from build123d import *

# Parameters (mm, degrees)
SKETCH1_W           = 200
SKETCH1_H           = 5
BOSS_EXTRUDE1_DEPTH = 5
SKETCH2_W           = 4.5
SKETCH2_H           = 5
CUT_EXTRUDE1_DEPTH  = 2.475
SKETCH3_R           = 2
BOSS_EXTRUDE3_DEPTH = 4.95
SKETCH4_R           = 2
BOSS_EXTRUDE4_DEPTH = 4.95


with BuildPart() as part:
    # Sketch1 → Boss-Extrude1 (new body)
    with BuildSketch(Plane.XY):
        with Locations((100, 2.5)):
            Rectangle(SKETCH1_W, SKETCH1_H)
    extrude(amount=BOSS_EXTRUDE1_DEPTH)

    # Sketch2 → Cut-Extrude1 (cut, symmetric)
    with BuildSketch(Plane.XY.offset(2.5)):
        with Locations((2.25, 2.5)):
            Rectangle(SKETCH2_W, SKETCH2_H)
        with Locations((197.75, 2.5)):
            Rectangle(SKETCH2_W, SKETCH2_H)
    extrude(amount=CUT_EXTRUDE1_DEPTH, both=True, mode=Mode.SUBTRACT)

    # Sketch3 → Boss-Extrude3 (add)
    with BuildSketch(Plane.XY.offset(0.025)):
        with Locations(Location((2, 2.5, 0), (0, 0, 180))):
            Circle(SKETCH3_R)
    extrude(amount=BOSS_EXTRUDE3_DEPTH)

    # Sketch4 → Boss-Extrude4 (add)
    with BuildSketch(Plane.XY.offset(0.025)):
        with Locations((198, 2.5)):
            Circle(SKETCH4_R)
    extrude(amount=BOSS_EXTRUDE4_DEPTH)


solid = part.part
Geometry check sheet. Reference: the model listing, model coordinates, mm. A direction names the side the tool comes from. Round coordinates to 2 decimals unless told otherwise and drop trailing zeros. Loops run counter-clockwise (first coordinate to the right, second up) from the corner with the lowest first, then second, coordinate; pieces in that order, holes last.
Item 1: Cross-section at B-B on x = 2. Record the boundary of the cut face in (y, z) (3 decimals), then the cut area to 4 significant figures.
Item 2: Cross-section at A-A on z = 2.8. Record the boundary of the cut face in (x, y), then the cut area to 3 significant figures.
Item 3: Mould release check, pull along Z, two halves, no side actions. Record for faces 4 (the flat face through (4.5, 2, 2)), 5 (the cylindrical face through (196.002, 2.588, 2.465)), 6 (the flat face through (99, 3, 0)), 7 (the flat face through (99, 3, 5)): pulls with the +Z half, pulls with the -Z half, needs draft (parallel to the pull), parting line crosses it, or undercut.
Item 4: Gauge pin test, flat ends, axial feed: pin 1 (2 mm diameter, centred on x = 35, z = 2.5, fed in from -Y); pin 2 (1 mm diameter, centred on y = 3.5, z = 1, fed in from -X). Record the tip position at first contact, or that the pin passes through.
Item 5: Thickness scan on line 1 (X direction, y = 2.7, z = 1.85); line 2 (X direction, y = 4.25, z = 0.7); line 3 (X direction, y = 0.35, z = 3.85). Record the ranges inside material, lowest first.
Item 6: Access from +Z, -Z, +X, -X, +Y, -Y to the whole of each face (thin tool, end or side, straight path). Record for faces 1 (the cylindrical face through (3.6, 3.7, 2.5)), 2 (the flat face through (99, 5, 2)), 3 (the flat face through (195.5, 2, 3)).
Answer sheet:
1. outline: (0, 0) - (5, 0) - (5, 0.025) - (4.5, 0.025) - (4.5, 4.975) - (5, 4.975) - (5, 5) - (0, 5) - (0, 4.975) - (0.5, 4.975) - (0.5, 0.025) - (0, 0.025) - close
1. area: 20.05 mm2
2. outline: circle Ø4 at (2, 2.5); (4.5, 0) - (195.5, 0) - (195.5, 5) - (4.5, 5) - close; circle Ø4 at (198, 2.5)
2. area: 980 mm2
3. face 4: undercut
3. face 5: undercut
3. face 6: pulls with the -Z half
3. face 7: pulls with the +Z half
4. pin 1: stops at y = 0
4. pin 2: stops at x = 0.06
5. line 1: x = 0.01 to 3.99, 4.5 to 195.5, 196.01 to 199.99
5. line 2: x = 1.03 to 2.97, 4.5 to 195.5, 197.03 to 198.97
5. line 3: x = 4.5 to 195.5
6. face 1: none
6. face 2: +Z, -Z, +X, -X, +Y
6. face 3: +Y, -Y
